Verification items for the finished model (mm, model axes). A direction names the side the tool comes from. Round coordinates to 2 decimals unless told otherwise and drop trailing zeros. Write each loop counter-clockwise with the first axis right and the second up, starting at its lowest first coordinate (ties: lowest second). Pieces come first, ordered by that corner, then holes. Notation, with made-up numbers: M 63.5,-6 L 115.5,-6 A16 cw 115.5,9 Z; hole C 64.25,-36 d7. An arc over 180 degrees is marked long. One line per item, written item: value. Start each with the question number.
from build123d import *

# Parameters (mm, degrees)
SKETCH_W                  = 80
SKETCH_H                  = 45
PAD_DEPTH                 = 1.7
SKETCH001_W               = 6.5
SKETCH001_H               = 11
PAD001_DEPTH              = 11.5
SKETCH002_W               = 6.5
SKETCH002_H               = 15
PAD002_DEPTH              = 11.5
SKETCH003_W               = 18.5
SKETCH003_H               = 15
PAD003_DEPTH              = 16.8
CYLINDER_R                = 1.5
CYLINDER_DEPTH            = 10
CYLINDER_MIRRORED_2_R     = 1.5
CYLINDER_MIRRORED_2_DEPTH = 10
SKETCH034_W               = 28
SKETCH034_H               = 38.5
PAD017_DEPTH              = 12
SKETCH035_W               = 22
SKETCH035_H               = 12.5
PAD018_DEPTH              = 15.5


with BuildPart() as part:
    # Sketch → Pad (new body)
    with BuildSketch(Plane.XY):
        Rectangle(SKETCH_W, SKETCH_H)
    extrude(amount=PAD_DEPTH)

    # Sketch001 → Pad001 (join)
    with BuildSketch(Plane.XY):
        with Locations((-36.75, 8.6)):
            Rectangle(SKETCH001_W, SKETCH001_H)
    extrude(amount=PAD001_DEPTH)

    # Sketch002 → Pad002 (join)
    with BuildSketch(Plane.XY):
        with Locations((-36.75, -8.5)):
            Rectangle(SKETCH002_W, SKETCH002_H)
    extrude(amount=PAD002_DEPTH)

    # Sketch003 → Pad003 (join)
    with BuildSketch(Plane.XY):
        with Locations((-19.75, -13)):
            Rectangle(SKETCH003_W, SKETCH003_H)
    extrude(amount=PAD003_DEPTH)

    # Cylinder → Cylinder (cut)
    with BuildSketch(Plane(origin=(37, 19.5, 0), x_dir=(1, 0, 0), z_dir=(0, 0, 1))):
        Circle(CYLINDER_R)
    cylinder = extrude(amount=CYLINDER_DEPTH, mode=Mode.SUBTRACT)

    # Cylinder Mirrored 2 → Cylinder Mirrored 2 (cut)
    with BuildSketch(Plane(origin=(-37, 19.5, 0), x_dir=(-1, 0, 0), z_dir=(0, 0, -1))):
        Circle(CYLINDER_MIRRORED_2_R)
    cylinder_mirrored_2 = extrude(amount=-CYLINDER_MIRRORED_2_DEPTH, mode=Mode.SUBTRACT)

    # Mirrored001: Cylinder, Cylinder Mirrored 2 across XZ
    add(cylinder.mirror(Plane.XZ), mode=Mode.SUBTRACT)
    add(cylinder_mirrored_2.mirror(Plane.XZ), mode=Mode.SUBTRACT)

    # Sketch034 → Pad017 (join)
    with BuildSketch(Plane.XY):
        with Locations((20, 0)):
            Rectangle(SKETCH034_W, SKETCH034_H)
    extrude(amount=PAD017_DEPTH)

    with BuildSketch(Plane(origin=(22, 4.5, 12), x_dir=(-1, 0, 0), z_dir=(0, 0, -1))):
        Rectangle(SKETCH035_W, SKETCH035_H)
    extrude(amount=-PAD018_DEPTH)


solid = part.part
1) Access from +Z, -Z, +X, -X, +Y, -Y to the whole of each face (thin tool, end or side, straight path). Record for faces 4 (the flat face through (11, 4, 20)), 5 (the flat face through (20, 19.25, 7)), 6 (the flat face through (33, 4, 20)), 7 (the flat face through (20, -19.25, 7)), 8 (the flat face through (6, 0, 7)).
2) Cross-section at B-B (z = 15.5). Record the boundary of the cut face in (x, y), then the cut area to 4 significant figures.
3) Mould release check, pull along X, two halves, no side actions. Record for faces 1 (the flat face through (-29, -13, 9)), 2 (the flat face through (-37, -16, 7)), 3 (the flat face through (40, 0, 1)): pulls with the +X half, pulls with the -X half, needs draft (parallel to the pull), parting line crosses it, or undercut.
4) Cross-section at C-C (y = 4.5). Record the boundary of the cut face in (x, z), then the cut area to 3 significant figures.
5) Cross-section at A-A (x = 37). Record the boundary of the cut face in (y, z), then the cut area to 3 significant figures.
6) Cross-section at D-D (x = 16). Record the boundary of the cut face in (y, z).
7) Gauge pin test, flat ends, axial feed: pin 1 Ø16.5 at (y, z) = (-15.5, 12) entering from +X; pin 2 Ø7.5 at (x, z) = (-20.5, 8.5) entering from -Y; pin 3 Ø8 at (x, y) = (0, -6) entering from +Z; pin 4 Ø12 at (x, y) = (19.5, 9.5) entering from -Z. Record the tip position at first contact, or that the pin passes through.
8) Thickness scan on line 1 (Y direction, x = 37, z = 0.95); line 2 (X direction, y = -9, z = 9.75); line 3 (X direction, y = -16.5, z = 6.25). Record the ranges inside material, lowest first.
Results below:
1. face 4: +Z, -X, +Y, -Y
1. face 5: +Z, +X, -X, +Y
1. face 6: +Z, +X, +Y, -Y
1. face 7: +Z, +X, -Y
1. face 8: +Z, +Y, -Y
2. outline: M -29,-20.5 L -10.5,-20.5 L -10.5,-5.5 L -29,-5.5 Z; M 11,-1.75 L 33,-1.75 L 33,10.75 L 11,10.75 Z
2. area: 552.5 mm²
3. face 1: undercut
3. face 2: needs draft
3. face 3: pulls with the +X half
4. outline: M -40,0 L 40,0 L 40,1.7 L 34,1.7 L 34,12 L 33,12 L 33,27.5 L 11,27.5 L 11,12 L 6,12 L 6,1.7 L -33.5,1.7 L -33.5,11.5 L -40,11.5 Z
4. area: 829 mm²
5. outline: M -22.5,0 L -21,0 L -21,1.7 L -22.5,1.7 Z; M -18,0 L 18,0 L 18,1.7 L -18,1.7 Z; M 21,0 L 22.5,0 L 22.5,1.7 L 21,1.7 Z
5. area: 66.3 mm²
6. outline: M -22.5,0 L 22.5,0 L 22.5,1.7 L 19.25,1.7 L 19.25,12 L 10.75,12 L 10.75,27.5 L -1.75,27.5 L -1.75,12 L -19.25,12 L -19.25,1.7 L -22.5,1.7 Z
7. pin 1: stops at x = 34
7. pin 2: stops at y = -20.5
7. pin 3: stops at z = 1.7
7. pin 4: stops at z = 0
8. line 1: y = -22.5 to -21, -18 to 18, 21 to 22.5
8. line 2: x = -40 to -33.5, -29 to -10.5, 6 to 34
8. line 3: x = -29 to -10.5, 6 to 34
